Could you check a few things on this model? Use its own coordinates, in mm. A direction names the side the tool comes from. Coordinates: 2 decimals unless noted, no trailing zeros. Write each loop counter-clockwise with the first axis right and the second up, starting at its lowest first coordinate (ties: lowest second). Pieces come first, ordered by that corner, then holes.
```python
from build123d import *

# Parameters (mm, degrees)
BOSS_EXTRUDE1_DEPTH = 25
SKETCH3_W           = 54
SKETCH3_H           = 121
BOSS_EXTRUDE2_DEPTH = 2


with BuildPart() as part:
    # Sketch1 → Boss-Extrude1 (new body)
    with BuildSketch(Plane.XY):
        Polygon((2.337959557, 2.176185102), (2.337959557, 121.176185102), (-22.662040443, 121.176185102), (-22.662040443, 119.176185102), (0.337959557, 119.176185102), (0.337959557, 0.176185102), (54.337959557, 0.176185102), (54.337959557, 119.176185102), (77.337959557, 119.176185102), (77.337959557, 121.176185102), (52.337959557, 121.176185102), (52.337959557, 2.176185102), align=None)
    extrude(amount=BOSS_EXTRUDE1_DEPTH)

    # Sketch3 → Boss-Extrude2 (add)
    with BuildSketch(Plane.XY.offset(25)):
        with Locations((27.337959557, 60.676185102)):
            Rectangle(SKETCH3_W, SKETCH3_H)
    extrude(amount=BOSS_EXTRUDE2_DEPTH)


solid = part.part
```
1. If we mould it in two halves opening along X, with no side actions, what happens to faces 5 (the face through (27, 63, 25)), 6 (the face through (2.338, 61, 12)), 7 (the face through (1, 70, 0))? For each: pulls with the +X half, pulls with the -X half, needs draft (parallel to the pull), parting line crosses it, or undercut.
Verdict:
face 5: undercut
face 6: undercut
face 7: needs draft
2. I want a section at B-B on x = 22.5. Please give me the cut outline in (y, z).
Verdict:
outline: (0.18, 0) - (2.18, 0) - (2.18, 25) - (121.18, 25) - (121.18, 27) - (0.18, 27) - close
3. For pin 1 (8 mm diameter, centred on y = 39.5, z = 20, fed in from -X); pin 2 (2 mm diameter, centred on x = 9, z = 20, fed in from +Y); pin 3 (15 mm diameter, centred on x = 27.5, y = 82.5, fed in from -Z); pin 4 (5 mm diameter, centred on x = -1.5, y = 99, fed in from +Z), each with a flat end and sliding along its axis, tell me the tip position at first contact or that it passes through.
Verdict:
pin 1: stops at x = 0.34
pin 2: stops at y = 2.18
pin 3: stops at z = 25
pin 4: stops at z = 27
4. I want a section at C-C on z = 16.5. Please give me the cut outline in (x, y), plus the area to 3 significant figures.
Verdict:
outline: (-22.66, 119.18) - (0.34, 119.18) - (0.34, 0.18) - (54.34, 0.18) - (54.34, 119.18) - (77.34, 119.18) - (77.34, 121.18) - (52.34, 121.18) - (52.34, 2.18) - (2.34, 2.18) - (2.34, 121.18) - (-22.66, 121.18) - close
area: 676 mm2
5. On a 3-axis mill with a long thin cutter (end or side, diameter ignored), from which of +Z, -Z, +X, -X, +Y, -Y can I reach the whole of each face in a straight line? I mean faces 1 (the face through (52.338, 63, 12)), 2 (the face through (66, 119.176, 12)), 3 (the face through (26.6, 121.176, 25.3)), 4 (the face through (-11, 119.176, 12)). Say none if no direction works.
Verdict:
face 1: -Z, +Y
face 2: +Z, -Z, +X, -Y
face 3: +Z, -Z, +X, -X, +Y
face 4: +Z, -Z, -X, -Y
6. Please list where these lines run through material, in increasing order: line 1 along X through (y, z) = (106, 8.75); line 2 along Z through (x, y) = (2.5, 87); line 3 along Y through (x, z) = (16.5, 10.75).
Verdict:
line 1: x = 0.34 to 2.34, 52.34 to 54.34
line 2: z = 25 to 27
line 3: y = 0.18 to 2.18
7. I want a section at D-D on x = -8. Please give me the cut outline in (y, z), plus the area to 3 significant figures.
Verdict:
outline: (119.18, 0) - (121.18, 0) - (121.18, 25) - (119.18, 25) - close
area: 50.0 mm2
8. I want a section at A-A on y = 63.5. Please give me the cut outline in (x, z), plus the area to 3 significant figures.
Verdict:
outline: (0.34, 0) - (2.34, 0) - (2.34, 25) - (52.34, 25) - (52.34, 0) - (54.34, 0) - (54.34, 27) - (0.34, 27) - close
area: 208 mm2
